Geometry check sheet. Reference: the model listing, model coordinates, mm. A direction names the side the tool comes from. Round coordinates to 2 decimals unless told otherwise and drop trailing zeros. Loops run counter-clockwise (first coordinate to the right, second up) from the corner with the lowest first, then second, coordinate; pieces in that order, holes last. Notation, with made-up numbers: (45.5, 24.5) - (49.5, 24.5) arc R10 cw to (49.5, 38.5) - close; hole circle Ø6 at (86.25, 3). An arc over 180 degrees is marked (long way). Write item = value, one per line.
Autodesk Fusion 360 part; units mm, degrees
sketch "Sketch1" plane through (0, 0, 0) normal (0, 0, 1) x (1, 0, 0)
  circle A0 centre (0, 0) radius 42.5
  circle A1 centre (0, 0) radius 46.5
  dimension "d1" = 85
  dimension "d2" = 93
extrude "Extrude1" add sketch "Sketch1" along normal blind 46 makes body 1
extrude "Extrude2" add sketch "Sketch1" against normal blind 4 contours A0 | A1 bodies 1
ref_plane "WorkPlane1" through (0, 0, 46) normal (0, 0, 1) x (1, 0, 0)
sketch "Sketch3" plane through (0, 0, 46) normal (0, 0, 1) x (1, 0, 0)
  circle A0 centre (0, 0) radius 46.5
  circle A1 centre (0, 0) radius 42.5
  circle A2 centre (0, 0) radius 49
  circle A3 centre (0, 0) radius 40.5
  circle A4 centre (0, 0) radius 46.9
  dimension "d9" = 98
  dimension "d10" = 81
  dimension "d50" = 0.4
extrude "Extrude3" add sketch "Sketch3" along normal blind 4 separate body contours A0 | A1 | A2 | A4 makes body 2
extrude "Extrude4" add sketch "Sketch3" against normal blind 12 contours A2 bodies 2
chamfer "Chamfer1" distance 3 angle 45 1 edges at (-37.7593, 14.6454, 50) on bodies 2
chamfer "Chamfer2" distance 2 angle 65 1 edges at (-45.684, -17.7192, 50) measured on face at (46.8223, -4.5955, 50) on bodies 2
chamfer "Chamfer3" distance 1 angle 45 1 edges at (-45.684, 17.7192, 34) measured on face at (48.1176, -2.4344, 34) on bodies 2
chamfer "Chamfer4" distance 1 angle 45 1 edges at (-43.3532, 16.8151, -4) measured on face at (10.204, -8.5364, -4) on bodies 1
ref_plane "WorkPlane2" through (0, 0, 0) normal (0, 0, -1) x (-1, 0, 0)
sketch "Sketch4" plane through (0, 0, 0) normal (0, 0, -1) x (1, 0, 0)
  circle A0 centre (0, 0) radius 46.5 construction
  line L0 (-37.4678, -27.5394) -> (-20.6148, -41.6807)
  line L1 (-20.6148, -41.6807) -> (-26.0712, -48.1834)
  line L2 (-26.0712, -48.1834) -> (-42.9242, -34.0421)
  line L3 (-42.9242, -34.0421) -> (-37.4678, -27.5394)
  line L4 (0, 0) -> (-58.0825, -69.2201) construction
  line L5 (-18.892, -39.6276) -> (-35.745, -25.4862)
  circle A1 centre (0, 0) radius 42.5
  line L6 (-18.892, -39.6276) -> (-8.0933, -41.7223)
  line L7 (-35.745, -25.4862) -> (-39.683, -15.2153)
  line L8 (-39.683, -15.2153) -> (-8.0933, -41.7223)
  line L9 (0, 0) -> (-65, 0) construction
  dimension "d26" = 22
  dimension "d58" = 50
extrude "Extrude5" cut sketch "Sketch4" along normal through all and the other way through all contours L0 L1 L2 L3 bodies 1
sketch "Sketch5" plane through (-29.0413, 34.61, 0) normal (-0.6428, 0.766, 0) x (-0.766, -0.6428, 0)
  line L0 (-11, 46) -> (-11, -3)
  circle A0 centre (0, 20) radius 6.5
  line L1 (11, 46) -> (-11, 46)
  spline S0 degree 2 poles (-5.3852, -4) (-8.1621, -3.6713) (-11, -3) knots 0 0 0 0.570553 0.570553 0.570553 weights 1 1.001868 1
  line L2 (-5.3852, -4) -> (5.3852, -4)
  spline S1 degree 2 poles (11, -3) (8.1621, -3.6713) (5.3852, -4) knots 0 0 0 0.570553 0.570553 0.570553 weights 1 1.001868 1
  line L3 (11, -3) -> (11, 46)
  line L4 (-11, 0) -> (11, 0)
  dimension "d30" = 13
  dimension "d61" = 20
  dimension "d62" = 11
extrude "Extrude6" cut sketch "Sketch5" along direction (0.707107, -0.707107, 0) blind 15 contours A0 bodies 1
sketch "Sketch6" plane through (0, 0, 0) normal (0, 0, 1) x (-1, 0, 0)
  circle A0 centre (0, -35) radius 3
  circle A1 centre (30.31, 17.5) radius 3
  circle A2 centre (-30.31, 17.5) radius 3
  circle A3 centre (0, 0) radius 5
  circle A4 centre (0, 0) radius 42.5
  circle A5 centre (20, 0) radius 2.75
  line L0 (0, 0) -> (65, 0)
  circle A6 centre (-20, 0) radius 2.75
  circle A7 centre (20, 0) radius 5
  circle A8 centre (-20, 0) radius 5
  dimension "d33" = 6
  dimension "d34" = 6
  dimension "d35" = 6
  dimension "d36" = 35
  dimension "d37" = 17.5
  dimension "d38" = 17.5
  dimension "d39" = 30.31
  dimension "d40" = 30.31
  dimension "d42" = 10
  dimension "d63" = 5.5
  dimension "d64" = 5.5
  dimension "d65" = 10
  dimension "d66" = 10
  dimension "d67" = 20
  dimension "d68" = 20
extrude "Extrude7" cut sketch "Sketch6" against normal through all contours A3 | A5 L0 | A5 L0 | A6 bodies 1
extrude "Extrude8" add sketch "Sketch6" along normal blind 2 contours A0 | A1 | A2 bodies 1
sketch "Sketch7" plane through (0, 0, 2) normal (0, 0, 1) x (-1, 0, 0)
  circle A0 centre (0, -35) radius 3
  circle A1 centre (0, -35) radius 1.5
  circle A2 centre (30.31, 17.5) radius 1.5
  circle A3 centre (-30.31, 17.5) radius 1.5
  point P0 (30.31, 17.5)
  point P1 (-30.31, 17.5)
  dimension "d45" = 3
  dimension "d46" = 3
  dimension "d47" = 3
extrude "Extrude9" cut sketch "Sketch7" against normal through all contours A1 | A2 | A3 bodies 1
chamfer "Chamfer5" distance 1 angle 45 1 edges at (-43.3532, -16.8151, 46) measured on face at (-19.1306, 39.3496, 46) on bodies 1
extrude "Extrude11" cut sketch "Sketch4" against normal through all contours L5 A1 L6 | L5 A1 L7 bodies 1
chamfer "Chamfer7" distance 1 angle 45 3 edges at (-13.4926, 40.6749, 0) (27.3185, -32.5569, 0) (-37.714, 20.3508, 0) on bodies 1
extrude "Extrude12" cut sketch "Sketch6" against normal blind 2 contours A5 L0 A7 | A5 L0 A7 | A8 bodies 1
chamfer "Chamfer8" distance 1 angle 45 2 edges at (-15.3384, -1.8081, 0) (24.6616, -1.8081, 0) on bodies 1
hidden bodies 2
(1) Scan lines: L1, parallel to Y at x = 0, z = -2.1; L2, parallel to Y at x = 0, z = 18; L3, parallel to X at y = -17.5, z = -1.7. Record each from-to range of solid material in increasing order. Write a range as [from, to].
Answers follow:
L1 = [-46.5, -5], [5, 33.5], [36.5, 46.5]
L2 = [-46.5, -42.5], [42.5, 46.5]
L3 = [-43.08, -31.81], [-28.81, 28.81], [31.81, 43.08]
(2) Set-up check for faces 1 (the cylindrical face through (24.995, -0.22, -1.493)), 2 (the cylindrical face through (28.418, -36.806, 21.336)): record each of +Z, -Z, +X, -X, +Y, -Y from which the full face is reachable in a straight line by a thin tool's end or side.
Answers follow:
face_1 = +Z
face_2 = +Z, -Z
(3) Mould release check, pull along X, two halves, no side actions. Record for faces 3 (the cylindrical face through (-28.81, -17.57, -0.96)), 4 (the flat face through (-29.16, 34.51, 26.91)), 5 (the flat face through (33.5, -26.8, 46)), 6 (the flat face through (9, 1, 0)): pulls with the +X half, pulls with the -X half, needs draft (parallel to the pull), parting line crosses it, or undercut.
Answers follow:
face_3 = undercut
face_4 = pulls with the -X half
face_5 = needs draft
face_6 = undercut
(4) Section check A-A (z = 36). Enter the section's corners in (x, y) (3 decimals), then the cut area to 3 significant figures.
Answers follow:
outline = (-37.468, 27.539) arc R46.5 ccw (long way) to (-20.615, 41.681) - close; hole (-39.683, 15.215) arc R42.5 ccw (long way) to (-8.093, 41.722) - (-18.892, 39.628) - (-35.745, 25.486) - close
area = 1,080 mm²
(5) Section check B-B (x = -30.5). State how many separate pieces and enclosed holes the cut face has, then the cut area to 3 significant figures.
Answers follow:
separate_pieces = 3
enclosed_holes = 0
area = 642 mm²
(6) Gauge pin test, flat ends, axial feed: pin 1 (1.5 mm diameter, centred on x = -14, z = 9.5, fed in from -Y); pin 2 (5 mm diameter, centred on x = 0, y = 35, fed in from +Z); pin 3 (11 mm diameter, centred on x = -18, y = 0, fed in from +Z); pin 4 (2.5 mm diameter, centred on x = 0, y = 35, fed in from -Z). Record the tip position at first contact, or that the pin passes through.
Answers follow:
pin_1 = -44.57
pin_2 = 2
pin_3 = 0
pin_4 = through
